The listing builds one solid part. Answer for the finished solid, in the listing's coordinates (mm). A direction names the side the tool comes from. Coordinates: 2 decimals unless noted, no trailing zeros. Order: outer loops, then holes, each group sorted by start corner. A loop starts at its lowest first (then second) coordinate and runs counter-clockwise, first axis right, second up. Notation, with made-up numbers: (41, 52) -> (94, 52) arc R26 ccw to (94, 82) -> close; hole circle Ø11 at (18, -22). An arc over 180 degrees is marked (long way). Answer in a Markdown table with one row per item. Add a question column.
Autodesk Inventor part; units mm, degrees
ref_plane "YZ Plane" through (0, 0, 0) normal (1, 0, 0) x (0, 1, 0)
ref_plane "XZ Plane" through (0, 0, 0) normal (0, 1, 0) x (-1, 0, 0)
ref_plane "XY Plane" through (0, 0, 0) normal (0, 0, 1) x (1, 0, 0)
ref_plane "Work Plane1" through (0, 0, 0) normal (0, 0, 1) x (1, 0, 0)
sketch "Sketch1" plane through (0, 0, 0) normal (0, 0, 1) x (1, 0, 0)
  circle A0 centre (0, 0) radius 11
  circle A1 centre (0, 0) radius 4
  circle A2 centre (0, 0) radius 37.5
  line L0 (0, 0) -> (0, 20) construction
  line L1 (0, 20) -> (-15, 20) construction
  line L2 (0, 20) -> (15, 20) construction
  line L3 (0, -2.0548) -> (-11.5, -2.0548) construction
  line L4 (0, -2.0548) -> (11.5, -2.0548) construction
  arc A3 (-11.5, -2.0548) -> (11.5, -2.0548) centre (0, 0.9175) ccw
  line L5 (-40, -40) -> (40, -40) construction
  line L6 (40, -40) -> (40, 40) construction
  line L7 (40, 40) -> (-40, 40) construction
  line L8 (-40, 40) -> (-40, -40) construction
  line L9 (-40, -40) -> (40, 40) construction
  line L10 (40, -40) -> (-40, 40) construction
  line L11 (0, 11) -> (0, 16) construction
  line L12 (0, 16) -> (13.8259, 16) construction
  line L13 (13.8259, 16) -> (40, 16)
  line L14 (-15, 20) -> (-15, 39)
  line L15 (-15, 39) -> (40, 39)
  line L16 (11.5, -2.0548) -> (13.8259, 16)
  line L17 (-15, 20) -> (-11.5, -2.0548)
  line L18 (-17, 41) -> (-17, 19.8423)
  line L19 (-17, 19.8423) -> (-13.4609, -2.459)
  arc A4 (-13.4609, -2.459) -> (13.4683, -2.4294) centre (0, 0.9175) ccw
  line L20 (13.4683, -2.4294) -> (15.5848, 14)
  line L21 (40, 39) -> (40, 41)
  line L22 (40, 16) -> (40, 14)
  line L23 (-17, 41) -> (40, 41)
  line L24 (40, 14) -> (15.5848, 14)
  point P0 (0, 0)
  dimension "d0" = 15
  dimension "d1" = 20
  dimension "d2" = 15
  dimension "d3" = 11.5
  dimension "d4" = 11.5
  dimension "d5" = 80
  dimension "d6" = 80
  dimension "d7" = 5
  dimension "d8" = 23
  dimension "d9" = 2
extrude "Extrusion1" add sketch "Sketch1" along normal blind 8 contours A0 A3 L16 L13 A2 L24 L20 A4 L19 L18 L14 L17 | A2 L18 L23 L21 L15 L14 | L13 L22 L24 A2
sketch "Sketch2" plane through (0, 0, 8) normal (0, 0, 1) x (1, 0, 0)
  line L0 (-42.5, 42.5) -> (42.5, 42.5)
  line L1 (42.5, 42.5) -> (42.5, -42.5)
  line L2 (42.5, -42.5) -> (-42.5, -42.5)
  line L3 (-42.5, -42.5) -> (-42.5, 42.5)
  line L4 (-42.5, 42.5) -> (42.5, -42.5) construction
  line L5 (42.5, 42.5) -> (-42.5, -42.5) construction
  point P0 (0, 0)
  dimension "d12" = 85
  dimension "d13" = 85
extrude "Extrusion2" add sketch "Sketch2" along normal blind 2
sketch "Sketch3" plane through (0, 0, 8) normal (0, 0, -1) x (-1, 0, 0)
  line L0 (-13.4683, -2.4294) -> (-15.5848, 14)
  arc A0 (-13.4683, -2.4294) -> (13.4609, -2.459) centre (0, 0.9175) ccw
  line L1 (17, 19.8423) -> (13.4609, -2.459)
  line L2 (17, 41) -> (17, 19.8423)
  line L3 (-40, 41) -> (17, 41)
  line L4 (-40, 39) -> (-40, 41)
  line L5 (15, 39) -> (-40, 39)
  line L6 (15, 20) -> (15, 39)
  line L7 (11.5, -2.0548) -> (15, 20)
  arc A1 (-11.5, -2.0548) -> (11.5, -2.0548) centre (0, 0.9175) ccw
  line L8 (-13.8259, 16) -> (-11.5, -2.0548)
  line L9 (-40, 16) -> (-13.8259, 16)
  line L10 (-40, 14) -> (-40, 16)
  line L11 (-15.5848, 14) -> (-40, 14)
  line L12 (42.5, 42.5) -> (42.5, -42.5)
  line L13 (-42.5, 42.5) -> (42.5, 42.5)
  line L14 (-42.5, -42.5) -> (-42.5, 42.5)
  line L15 (42.5, -42.5) -> (-42.5, -42.5)
  arc A2 (-13.4683, -2.4294) -> (13.4609, -2.459) centre (0, 0.9175) ccw
  line L16 (-13.4683, -2.4294) -> (-15.5848, 14)
  line L17 (-15.5848, 14) -> (-40, 14)
  line L18 (-40, 14) -> (-40, 16)
  line L19 (-40, 16) -> (-13.8259, 16)
  line L20 (-13.8259, 16) -> (-11.5, -2.0548)
  arc A3 (-11.5, -2.0548) -> (11.5, -2.0548) centre (0, 0.9175) ccw
  line L21 (11.5, -2.0548) -> (15, 20)
  line L22 (15, 20) -> (15, 39)
  line L23 (15, 39) -> (-40, 39)
  line L24 (-40, 39) -> (-40, 41)
  line L25 (-40, 41) -> (17, 41)
  line L26 (17, 41) -> (17, 19.8423)
  line L27 (17, 19.8423) -> (13.4609, -2.459)
  line L28 (42.5, -42.5) -> (-42.5, -42.5)
  line L29 (-42.5, 42.5) -> (42.5, 42.5)
  line L30 (42.5, 42.5) -> (42.5, -42.5)
  line L31 (42.5, -42.5) -> (-42.5, -42.5)
  line L32 (-42.5, -42.5) -> (-42.5, 42.5) construction
  line L33 (41, 41) -> (-41, 41)
  line L34 (-41.25, -41) -> (41, -41)
  line L35 (41, -41) -> (41, 41)
  line L36 (-40, 14) -> (-40, 16)
  line L37 (-40, 16) -> (-42.5, 16)
  line L38 (-15.5848, 14) -> (-40, 14)
  line L39 (-40, 14) -> (-42.5, 14)
  line L40 (-40, 39) -> (-42.5, 39)
  line L41 (-40, 41) -> (17, 41)
  line L42 (-40, 41) -> (-42.5, 41)
  line L43 (-41.25, -41) -> (-41.25, 14)
  line L44 (-42.5, -42.5) -> (-42.5, 42.5)
  line L45 (-42.5, -42.5) -> (-42.5, 14)
  line L46 (-40, 41) -> (17, 41)
  line L47 (-42.5, 41) -> (-42.5, 39)
  line L48 (41, 41) -> (41, 42.5)
  line L49 (-42.5, 42.5) -> (42.5, 42.5)
  point P0 (0, 0)
  dimension "d16" = 1.5
  dimension "d19" = 1.5
extrude "Extrusion4" add sketch "Sketch3" along normal blind 115 contours L39 L14 L37 L10 | L43 L34 L35 L48 L13 L12 L15 L14 L39
sketch "Sketch4" plane through (-42.5, -42.5, 10) normal (0, -1, 0) x (1, 0, 0)
  line L0 (78, -15) -> (72, -15)
  line L1 (70, -17) -> (70, -58)
  line L2 (72, -60) -> (78, -60)
  line L3 (80, -58) -> (80, -17)
  line L4 (0, 0) -> (85, 0)
  line L5 (85, -117) -> (85, 0)
  arc A0 (80, -17) -> (78, -15) centre (78, -17) ccw
  arc A1 (78, -60) -> (80, -58) centre (78, -58) ccw
  arc A2 (70, -58) -> (72, -60) centre (72, -58) ccw
  arc A3 (72, -15) -> (70, -17) centre (72, -17) ccw
  point P0 (42.5, -10)
  dimension "d22" = 15
  dimension "d23" = 5
  dimension "d24" = 15
  dimension "d25" = 60
  dimension "d26" = 2
extrude "Extrusion5" cut sketch "Sketch4" against normal through all
properties part number "Mount"
Q1. For faces 5 (the face through (12, 39, 4)), 6 (the face through (-13.274, 9.127, 3.944)), 7 (the face through (-17, 31, 4)), determine the directions among +Z, -Z, +X, -X, +Y, -Y from which every point of the face is accessible in a straight line to the end or side of a thin tool.
Q2. A cutting plane is placed at A-A (z = -44.5). Determine the outline of the cut face in (x, y), then the cut area to 4 significant figures.
Q3. Determine the mould class of faces 1 (the face through (1, -42.5, -49)), 2 (the face through (13.5, 12.1, 0)), 3 (the face through (-15, 29, 4)), 4 (the face through (0, 1, 8)) for opening direction Y: +Y half, -Y half, draft (parallel to the pull), parting line (faces both ways), or undercut.
Q4. Given pin 1 (9 mm diameter, centred on x = 6.5, z = 2.5, fed in from +Y); pin 2 (2 mm diameter, centred on y = 40.5, z = 5, fed in from +X), each flat-ended and moving along its own axis, determine where each tip first touches the part or whether it passes through.
Q5. A cutting plane is placed at B-B (y = 22.5). Determine the outline of the cut face in (x, z), then the cut area to 4 significant figures.
Q6. A cutting plane is placed at C-C (x = 18). Determine the outline of the cut face in (y, z), then the cut area to 4 significant figures.
Q7. A cutting plane is placed at D-D (z = -96). Determine the outline of the cut face in (x, y).
Q8. Straight lines are drawn through the part: line 1 (Y direction, x = 29.5, z = 0.5); line 2 (X direction, y = -39, z = -88); line 3 (Z direction, x = -38, y = -32.5). For each, find the intervals that lie inside material, in ascending order.
Returned:
| question | item | result |
|---|---|---|
| 1 | face 5 | -Z, +X |
| 1 | face 6 | -Z |
| 1 | face 7 | -Z, +Y |
| 2 | outline | (-42.5, -42.5) -> (27.5, -42.5) -> (27.5, -41) -> (-41, -41) -> (-41, 42.5) -> (-42.5, 42.5) -> close; (37.5, -42.5) -> (42.5, -42.5) -> (42.5, 16) -> (40, 16) -> (40, 14) -> (41.25, 14) -> (41.25, -41) -> (37.5, -41) -> close |
| 2 | area | 311.5 mm² |
| 3 | face 1 | -Y half |
| 3 | face 2 | draft |
| 3 | face 3 | undercut |
| 3 | face 4 | undercut |
| 4 | pin 1 | stops at y = 41 |
| 4 | pin 2 | stops at x = 40 |
| 5 | outline | (-42.5, -107) -> (-41, -107) -> (-41, 8) -> (-17, 8) -> (-17, 0) -> (-15, 0) -> (-15, 8) -> (42.5, 8) -> (42.5, 10) -> (-42.5, 10) -> close |
| 5 | area | 358.5 mm² |
| 6 | outline | (-42.5, -107) -> (-41, -107) -> (-41, 8) -> (14, 8) -> (14, 0) -> (16, 0) -> (16, 8) -> (39, 8) -> (39, 0) -> (41, 0) -> (41, 8) -> (42.5, 8) -> (42.5, 10) -> (-42.5, 10) -> close |
| 6 | area | 374.5 mm² |
| 7 | outline | (-42.5, -42.5) -> (42.5, -42.5) -> (42.5, 16) -> (40, 16) -> (40, 14) -> (41.25, 14) -> (41.25, -41) -> (-41, -41) -> (-41, 42.5) -> (-42.5, 42.5) -> close |
| 8 | line 1 | y = -42.5 to -41, 14 to 16, 39 to 41 |
| 8 | line 2 | x = -42.5 to -41, 41.25 to 42.5 |
| 8 | line 3 | z = 8 to 10 |
